Read the model definition and answer for the solid it produces. Units are mm, in the model's axes. A direction names the side the tool comes from. Round coordinates to 2 decimals unless told otherwise and drop trailing zeros. Order: outer loops, then holes, each group sorted by start corner. A loop starts at its lowest first (then second) coordinate and runs counter-clockwise, first axis right, second up. Notation, with made-up numbers: (-24, 74.25) - (-10, 74.25) arc R15 cw to (-10, 85.25) - close; hole circle Ø10 at (-34.5, -8). An arc over 180 degrees is marked (long way). Put each result on its own line as item: value. Start each with the question number.
Q1. Each of these flat-tipped pins is pushed along its axis until it touches: pin 1 Ø3 at (x, y) = (19.5, 107.5) entering from +Z; pin 2 Ø8 at (x, y) = (21.5, 29) entering from +Z (3 decimals); pin 3 Ø3 at (x, z) = (20, -76) entering from +Y; pin 4 Ø2 at (x, z) = (37.5, -45) entering from +Y. Where does it stop, or does it pass through?
Q2. Which of the six approach directions +Z, -Z, +X, -X, +Y, -Y give full straight-line access (tool end or side, diameter ignored) to faces 4 (the face through (18, 62, -71)), 5 (the face through (36.69, 124.01, -46.55))?
Q3. Section C-C on z = -35.5 is taken. Give the vertices of the cut face in (x, y).
Q4. Find the intervals of material crossed by line 1 along Y through (x, z) = (15.5, -11.5); line 2 along X through (y, z) = (57.5, -21); line 3 along Z through (x, y) = (37, 1), in increasing order. Write a range as from..to.
Q5. Section A-A on x = 37.5 is taken. Give the vertices of the cut face in (y, z).
Q6. Section D-D on y = 29.5 is taken. Give the vertices of the cut face in (x, z), then the cut area to 3 significant figures.
Q7. For a pull along Y with two mould halves and no side action, classify faces 1 (the face through (0.348, 61.695, -54.832)), 2 (the face through (1, 2, -26)), 3 (the face through (2.86, 2.9, -26.2)) as pulls with the +Y half, pulls with the -Y half, needs draft (parallel to the pull), parting line crosses it, or undercut.
Q8. Section B-B on z = -45 is taken. Give the vertices of the cut face in (x, y), then the cut area to 3 significant figures.
Autodesk Fusion 360 part; units mm, degrees
sketch "Sketch1" plane through (0, 0, 0) normal (0, 1, 0) x (1, 0, 0)
  line L0 (0, 0) -> (50, 0)
  line L1 (50, 0) -> (50, 55)
  line L2 (50, 55) -> (0, 55)
  line L3 (0, 55) -> (0, 0)
  line L4 (50, 55) -> (50, 90)
  line L5 (50, 90) -> (33.3333, 90)
  line L6 (33.3333, 90) -> (0, 55)
  line L7 (28, 76) -> (28, -7.4569) construction
  point P0 (28, 84.4)
  dimension "d1" = 50
  dimension "d2" = 55
  dimension "d3" = 35
  dimension "d4" = 16.6667
  dimension "d17" = 22
extrude "Extrude1" add sketch "Sketch1" along normal blind 125
fillet "Fillet1" radius 5 1 edges at (0, 125, -27.5)
fillet "Fillet2" radius 5 1 edges at (0, 0, -27.5)
fillet "Fillet3" radius 5 7 edges at (19.1667, 125, -75.125) (1.4645, 123.5355, -56.5377) (0, 62.5, -55) (1.4645, 1.4645, -56.5377) (19.1667, 0, -75.125) (41.6667, 125, -90) (41.6667, 0, -90)
fillet "Fillet4" radius 5 3 edges at (33.961, 1.4645, -88.5355) (33.3333, 62.5, -90) (33.961, 123.5355, -88.5355)
shell "Shell1" thickness 2 removed faces 2 at (50, 43.3333, -30) at (33.3333, 81.6667, 0)
sketch "Sketch2" plane through (0, 125, 0) normal (0, 1, 0) x (-1, 0, 0)
  line L0 (-50, -85) -> (-35.4762, -85)
  line L1 (-35.4762, -85) -> (-5, -53)
  line L2 (-5, -53) -> (-5, 0)
  line L3 (-5, 0) -> (-50, 0)
  line L4 (-50, 0) -> (-50, -85)
  line L5 (0, 0) -> (-50, 0)
  line L6 (-5, -53) -> (0, -53)
  circle A0 centre (-37.5, -45) radius 1.75
  dimension "d12" = 3.5
  dimension "d13" = 12.5
  dimension "d16" = 45
extrude "Extrude2" cut sketch "Sketch2" against normal up to surface (125 mm away) contours A0
equation "d4 = d1 / 3"
Findings:
1. pin 1: z = -71
1. pin 2: z = -70.475
1. pin 3: y = 123.57
1. pin 4: through
2. face 4: +Z, +X
2. face 5: +Y, -Y
3. outline: (0, 5) arc R5 ccw to (5, 0) - (50, 0) - (50, 2) - (5, 2) arc R3 cw to (2, 5) - (2, 120) arc R3 cw to (5, 123) - (50, 123) - (50, 125) - (5, 125) arc R5 ccw to (0, 120) - close
4. line 1: 0..2, 123..125
4. line 2: 0..2
4. line 3: -88..-46.68, -43.32..0
5. outline: (0, -85) arc R5 ccw to (5, -90) - (120, -90) arc R5 ccw to (125, -85) - (125, -46.75) - (123, -46.75) - (123, -85) arc R3 cw to (120, -88) - (5, -88) arc R3 cw to (2, -85) - (2, -46.75) - (0, -46.75) - close; (0, -43.25) - (2, -43.25) - (2, 0) - (0, 0) - close; (123, -43.25) - (125, -43.25) - (125, 0) - (123, 0) - close
6. outline: (0, -53) arc R5 ccw to (1.38, -56.45) - (31.86, -88.45) arc R5 ccw to (35.48, -90) - (50, -90) - (50, -88) - (35.48, -88) arc R3 cw to (33.3, -87.07) - (2.83, -55.07) arc R3 cw to (2, -53) - (2, 0) - (0, 0) - close
6. area: 236 mm2
7. face 1: needs draft
7. face 2: pulls with the -Y half
7. face 3: undercut
8. outline: (0, 5) arc R5 ccw to (5, 0) - (35.75, 0) - (35.75, 2) - (5, 2) arc R3 cw to (2, 5) - (2, 120) arc R3 cw to (5, 123) - (35.75, 123) - (35.75, 125) - (5, 125) arc R5 ccw to (0, 120) - close; (39.25, 0) - (50, 0) - (50, 2) - (39.25, 2) - close; (39.25, 123) - (50, 123) - (50, 125) - (39.25, 125) - close
8. area: 421 mm2
